from build123d import *

# Parameters (mm, degrees)
SKETCH1_W           = 3
SKETCH1_H           = 20
SKETCH1_W_2         = 20
SKETCH1_H_2         = 3
BOSS_EXTRUDE1_DEPTH = 3


with BuildPart() as part:
    # Sketch1 → Boss-Extrude1 (new body)
    # profile 1 of 5: a face of its own
    with BuildSketch(Plane.XY):
        with Locations((-63.5, 0)):
            Rectangle(SKETCH1_W, SKETCH1_H)
    # profile 2 of 5: a face of its own
    with BuildSketch(Plane.XY):
        Polygon((10, -22.5), (62, -22.5), (62, -10), (62, 10), (62, 22.5), (38.3, 22.5), (38.3, 19.5), (39.65, 19.5), (39.65, 17), (38.3, 17), (38.3, 12.5), (35, 12.5), (35, 17), (33.65, 17), (33.65, 19.5), (35, 19.5), (35, 22.5), (10, 22.5), (-10, 22.5), (-35, 22.5), (-35, 19.5), (-33.65, 19.5), (-33.65, 17), (-35, 17), (-35, 12.5), (-38.3, 12.5), (-38.3, 17), (-39.65, 17), (-39.65, 19.5), (-38.3, 19.5), (-38.3, 22.5), (-62, 22.5), (-62, 10), (-62, -10), (-62, -22.5), (-10, -22.5), align=None)
        with BuildLine():
            ThreePointArc((-44, -5), (-48, -9), (-52, -5))
            Line((-52, -5), (-52, 5))
            ThreePointArc((-52, 5), (-48, 9), (-44, 5))
            Line((-44, 5), (-44, -5))
        make_face(mode=Mode.SUBTRACT)
        with BuildLine():
            ThreePointArc((-29, -5), (-33, -9), (-37, -5))
            Line((-37, -5), (-37, 5))
            ThreePointArc((-37, 5), (-33, 9), (-29, 5))
            Line((-29, 5), (-29, -5))
        make_face(mode=Mode.SUBTRACT)
        with BuildLine():
            ThreePointArc((-14, -5), (-18, -9), (-22, -5))
            Line((-22, -5), (-22, 5))
            ThreePointArc((-22, 5), (-18, 9), (-14, 5))
            Line((-14, 5), (-14, -5))
        make_face(mode=Mode.SUBTRACT)
        with BuildLine():
            Line((22, 5), (22, -5))
            ThreePointArc((22, -5), (18, -9), (14, -5))
            Line((14, -5), (14, 5))
            ThreePointArc((14, 5), (18, 9), (22, 5))
        make_face(mode=Mode.SUBTRACT)
        with BuildLine():
            Line((37, 5), (37, -5))
            ThreePointArc((37, -5), (33, -9), (29, -5))
            Line((29, -5), (29, 5))
            ThreePointArc((29, 5), (33, 9), (37, 5))
        make_face(mode=Mode.SUBTRACT)
        with BuildLine():
            Line((52, 5), (52, -5))
            ThreePointArc((52, -5), (48, -9), (44, -5))
            Line((44, -5), (44, 5))
            ThreePointArc((44, 5), (48, 9), (52, 5))
        make_face(mode=Mode.SUBTRACT)
    # profile 3 of 5: a face of its own
    with BuildSketch(Plane.XY):
        with Locations((0, 24)):
            Rectangle(SKETCH1_W_2, SKETCH1_H_2)
    # profile 4 of 5: a face of its own
    with BuildSketch(Plane.XY):
        with Locations((63.5, 0)):
            Rectangle(SKETCH1_W, SKETCH1_H)
    # profile 5 of 5: a face of its own
    with BuildSketch(Plane.XY):
        with Locations((0, -24)):
            Rectangle(SKETCH1_W_2, SKETCH1_H_2)
    extrude(amount=BOSS_EXTRUDE1_DEPTH)


solid = part.part
Part model, mm, in its own coordinate system. A direction names the side the tool comes from. Round coordinates to 2 decimals unless told otherwise and drop trailing zeros. Write each loop counter-clockwise with the first axis right and the second up, starting at its lowest first coordinate (ties: lowest second). Pieces come first, ordered by that corner, then holes. Notation, with made-up numbers: M 84.25,52 L 101.25,52 A11 cw 101.25,69 Z; hole C 88,66 d5. An arc over 180 degrees is marked long. Return JSON: item names as keys, results as strings. Group by question number.
(1) Two-plate mould, pull along X, no slides. Class faces 6 (the face through (65, 0, 1)), 7 (the face through (36, -22.5, 1)), 8 (the face through (-35, 21, 1)): +X half, -X half, draft (parallel to the pull), parting line (faces both ways), or undercut.
(2) Saw through at A-A on x = -48. Write the cut outline in (y, z), then the cut area to 3 significant figures.
(3) Saw through at B-B on y = 21. Write the cut outline in (x, z).
(4) Saw through at C-C on z = 1.5. Count the separate pieces of the cut face and the enclosed holes in it, then the cut area to 3 significant figures.
(5) Drill centre lines: probe 1 along Y at (x, z) = (-25.5, 1.5); probe 2 along X at (y, z) = (11.5, 1.7); probe 3 along Y at (x, z) = (-50, 2.85). Where is each one in solid material? Low to high.
(6) Saw through at D-D on x = 31.5. Write the cut outline in (y, z), then the cut area to 3 significant figures.
(7) Which spindle directions (+Z, -Z, +X, -X, +Y, -Y) get a long thin tool onto all of the face, cutting with end or side? Do faces 1 (the face through (0, 25.5, 1)), 2 (the face through (-52, 0, 1)), 3 (the face through (35, 15, 1)), 4 (the face through (-64, -10, 1)), 5 (the face through (63, 10, 1)). Say none if no direction does.
(8) Pin check, flat tips, straight feed: pin 1 Ø0.8 at (y, z) = (18, 1) entering from +X; pin 2 Ø1.5 at (x, z) = (38.5, 2) entering from -Y; pin 3 Ø1.5 at (y, z) = (15.5, 1) entering from -X. Stop position of each tip, or through.
Returned:
{
 "1": {"face 6": "+X half", "face 7": "draft", "face 8": "undercut"},
 "2": {"outline": "M -22.5,0 L -9,0 L -9,3 L -22.5,3 Z; M 9,0 L 22.5,0 L 22.5,3 L 9,3 Z", "area": "81.0 mm²"},
 "3": {"outline": "M -62,0 L -38.3,0 L -38.3,3 L -62,3 Z; M -35,0 L 35,0 L 35,3 L -35,3 Z; M 38.3,0 L 62,0 L 62,3 L 38.3,3 Z"},
 "4": {"separate pieces": "1", "enclosed holes": "6", "area": "4,960 mm²"},
 "5": {"probe 1": "-22.5 to 22.5", "probe 2": "-62 to 62", "probe 3": "-22.5 to -8.46, 8.46 to 22.5"},
 "6": {"outline": "M -22.5,0 L -8.71,0 L -8.71,3 L -22.5,3 Z; M 8.71,0 L 22.5,0 L 22.5,3 L 8.71,3 Z", "area": "82.8 mm²"},
 "7": {"face 1": "+Z, -Z, +X, -X, +Y", "face 2": "+Z, -Z", "face 3": "+Z, -Z, +Y", "face 4": "+Z, -Z, -X, -Y", "face 5": "+Z, -Z, +X, +Y"},
 "8": {"pin 1": "x = 62", "pin 2": "y = -22.5", "pin 3": "x = -62"}
}
